from build123d import *

# Parameters (mm, degrees)
EXTRUDE_1_DEPTH     = 145
SKETCH_2_R          = 1.35
CUT_EXTRUDE_1_DEPTH = 3
CUT_EXTRUDE_2_DEPTH = 2.5
CUT_EXTRUDE_3_DEPTH = 70
FILLET_1_R          = 2.5
FILLET_2_R          = 1.5


with BuildPart() as part:
    # 草图1 → 凸台-拉伸1 (new body)
    with BuildSketch(Plane.XY):
        Polygon((-13, -35.966337082), (-13, -23.466337082), (40.5, -23.466337082), (40.5, -93.466337082), (-13, -93.466337082), (-13, -80.966337082), (-10, -80.966337082), (-10, -90.966337082), (38, -90.966337082), (38, -25.966337082), (-10, -25.966337082), (-10, -35.966337082), align=None)
    extrude(amount=-EXTRUDE_1_DEPTH)

    # 草图2 → 切除-拉伸1 (cut)
    with BuildSketch(Plane.ZY.offset(13)):
        with Locations((-112.5, -30.966337082)):
            Circle(SKETCH_2_R)
        with Locations((-72.5, -30.966337082)):
            Circle(SKETCH_2_R)
        with Locations((-32.5, -30.966337082)):
            Circle(SKETCH_2_R)
        with Locations((-32.5, -85.966337082)):
            Circle(SKETCH_2_R)
        with Locations((-72.5, -85.966337082)):
            Circle(SKETCH_2_R)
        with Locations((-112.5, -85.966337082)):
            Circle(SKETCH_2_R)
    extrude(amount=-CUT_EXTRUDE_1_DEPTH, mode=Mode.SUBTRACT)

    # 草图3 → 切除-拉伸2 (cut)
    with BuildSketch(Plane.ZY.offset(-38)):
        with BuildLine():
            Line((-128, -33.466337082), (-83, -33.466337082))
            ThreePointArc((-83, -33.466337082), (-78, -38.466337082), (-83, -43.466337082))
            Line((-83, -43.466337082), (-128, -43.466337082))
            ThreePointArc((-128, -43.466337082), (-133, -38.466337082), (-128, -33.466337082))
        make_face()
        with BuildLine():
            Line((-128, -53.466337082), (-83, -53.466337082))
            ThreePointArc((-83, -53.466337082), (-78, -58.466337082), (-83, -63.466337082))
            Line((-83, -63.466337082), (-128, -63.466337082))
            ThreePointArc((-128, -63.466337082), (-133, -58.466337082), (-128, -53.466337082))
        make_face()
        with BuildLine():
            Line((-128, -73.466337082), (-83, -73.466337082))
            ThreePointArc((-83, -73.466337082), (-78, -78.466337082), (-83, -83.466337082))
            Line((-83, -83.466337082), (-128, -83.466337082))
            ThreePointArc((-128, -83.466337082), (-133, -78.466337082), (-128, -73.466337082))
        make_face()
        with BuildLine():
            Line((-60, -33.466337082), (-15, -33.466337082))
            ThreePointArc((-15, -33.466337082), (-10, -38.466337082), (-15, -43.466337082))
            Line((-15, -43.466337082), (-60, -43.466337082))
            ThreePointArc((-60, -43.466337082), (-65, -38.466337082), (-60, -33.466337082))
        make_face()
        with BuildLine():
            Line((-60, -53.466337082), (-15, -53.466337082))
            ThreePointArc((-15, -53.466337082), (-10, -58.466337082), (-15, -63.466337082))
            Line((-15, -63.466337082), (-60, -63.466337082))
            ThreePointArc((-60, -63.466337082), (-65, -58.466337082), (-60, -53.466337082))
        make_face()
        with BuildLine():
            Line((-60, -73.466337082), (-15, -73.466337082))
            ThreePointArc((-15, -73.466337082), (-10, -78.466337082), (-15, -83.466337082))
            Line((-15, -83.466337082), (-60, -83.466337082))
            ThreePointArc((-60, -83.466337082), (-65, -78.466337082), (-60, -73.466337082))
        make_face()
    extrude(amount=-CUT_EXTRUDE_2_DEPTH, mode=Mode.SUBTRACT)

    # 草图4 → 切除-拉伸3 (cut)
    with BuildSketch(Plane(origin=(0, -23.466337082, 0), x_dir=(1, 0, 0), z_dir=(0, 1, 0))):
        Polygon((28.75, 85.438393953), (-1.25, 72.5), (28.75, 59.561606047), align=None)
        Polygon((-1.25, 127.5), (28.75, 114.561606047), (28.75, 127.5), align=None)
        Polygon((-1.25, 112.938393953), (28.75, 100), (-1.25, 87.061606047), align=None)
        Polygon((-1.25, 57.938393953), (28.75, 45), (-1.25, 32.061606047), align=None)
        Polygon((-1.25, 17.5), (28.75, 30.438393953), (28.75, 17.5), align=None)
    extrude(amount=-CUT_EXTRUDE_3_DEPTH, mode=Mode.SUBTRACT)

    # 圆角1
    fillet_1_edges = [part.edges().sort_by_distance(p)[0] for p in [
        (-1.25, -92.216337082, -127.5),
        (28.75, -92.216337082, -127.5),
        (28.75, -92.216337082, -114.561606047),
        (-1.25, -24.716337082, -127.5),
        (28.75, -24.716337082, -127.5),
        (28.75, -24.716337082, -114.561606047),
        (-1.25, -92.216337082, -32.061606047),
        (-1.25, -92.216337082, -57.938393953),
        (28.75, -92.216337082, -45),
        (-1.25, -24.716337082, -32.061606047),
        (-1.25, -24.716337082, -57.938393953),
        (28.75, -24.716337082, -45),
        (-1.25, -92.216337082, -87.061606047),
        (-1.25, -92.216337082, -112.938393953),
        (28.75, -92.216337082, -100),
        (-1.25, -24.716337082, -87.061606047),
        (-1.25, -24.716337082, -112.938393953),
        (28.75, -24.716337082, -100),
        (28.75, -92.216337082, -85.438393953),
        (28.75, -92.216337082, -59.561606047),
        (-1.25, -92.216337082, -72.5),
        (28.75, -24.716337082, -85.438393953),
        (28.75, -24.716337082, -59.561606047),
        (-1.25, -24.716337082, -72.5),
        (28.75, -92.216337082, -17.5),
        (-1.25, -92.216337082, -17.5),
        (28.75, -92.216337082, -30.438393953),
        (28.75, -24.716337082, -17.5),
        (-1.25, -24.716337082, -17.5),
        (28.75, -24.716337082, -30.438393953),
    ]]
    fillet(fillet_1_edges, radius=FILLET_1_R)

    # 圆角2
    fillet_2_edges = [part.edges().sort_by_distance(p)[0] for p in [
        (-13, -23.466337082, -72.5),
        (40.5, -23.466337082, -72.5),
        (40.5, -93.466337082, -72.5),
        (-13, -93.466337082, -72.5),
        (-10, -90.966337082, -72.5),
        (38, -90.966337082, -72.5),
        (38, -25.966337082, -72.5),
        (-10, -25.966337082, -72.5),
    ]]
    fillet(fillet_2_edges, radius=FILLET_2_R)


solid = part.part
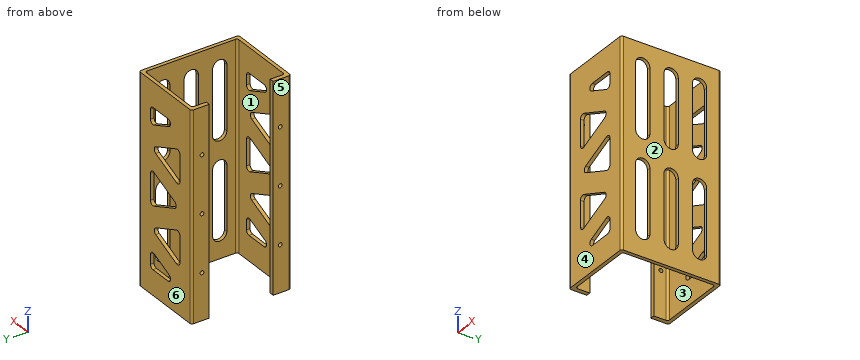
CAD build for the part. Positions are in the model's coordinates, mm. Face numbers are marked on the shaded views. A direction names the side the tool comes from. Give positions to 0.01 mm unless a question says otherwise; leave off trailing zeros. Order: outer loops, then holes, each group sorted by start corner. A loop starts at its lowest first (then second) coordinate and runs counter-clockwise, first axis right, second up. Notation, with made-up numbers: (45, -17) -> (85, -17) arc R17 cw to (85, -8) -> close; hole circle Ø6 at (55, 59.25). An arc over 180 degrees is marked (long way). Return JSON: item names as keys, results as strings.
Q1. Drill centre lines: line 1 (Y direction, x = -11, z = -72.5); line 2 (Y direction, x = -3.5, z = -46); line 3 (Y direction, x = -12, z = -72.5). Where is each one in solid material? Low to high.
Working result:
{"line 1": "-93.47 to -87.32, -84.62 to -80.97, -35.97 to -32.32, -29.62 to -23.47", "line 2": "-93.47 to -90.97, -25.97 to -23.47", "line 3": "-93.38 to -87.32, -84.62 to -80.97, -35.97 to -32.32, -29.62 to -23.55"}
Q2. Saw through at C-C (z = -135). Write the cut outline in (x, y), then the cut area to 3 significant figures.
Working result:
{"outline": "(-13, -91.97) arc R1.5 ccw to (-11.5, -93.47) -> (39, -93.47) arc R1.5 ccw to (40.5, -91.97) -> (40.5, -24.97) arc R1.5 ccw to (39, -23.47) -> (-11.5, -23.47) arc R1.5 ccw to (-13, -24.97) -> (-13, -35.97) -> (-10, -35.97) -> (-10, -27.47) arc R1.5 cw to (-8.5, -25.97) -> (36.5, -25.97) arc R1.5 cw to (38, -27.47) -> (38, -89.47) arc R1.5 cw to (36.5, -90.97) -> (-8.5, -90.97) arc R1.5 cw to (-10, -89.47) -> (-10, -80.97) -> (-13, -80.97) -> close", "area": "490 mm²"}
Q3. Saw through at A-A (x = -4). Write the cut outline in (y, z).
Working result:
{"outline": "(-93.47, -145) -> (-90.97, -145) -> (-90.97, 0) -> (-93.47, 0) -> close; (-25.97, -145) -> (-23.47, -145) -> (-23.47, 0) -> (-25.97, 0) -> close"}
Q4. Flat gauge pin, fed straight in: pin 1 (10 mm diameter, centred on y = -63.5, z = -72, fed in from -X). Where does the tip first touch, or does it go through?
Working result:
{"pin 1": "x = 38"}
Q5. Saw through at D-D (z = -104). Count the separate pieces of the cut face and the enclosed holes in it, then the cut area to 3 significant figures.
Working result:
{"separate pieces": "6", "enclosed holes": "0", "area": "311 mm²"}
Q6. Mould opens along Y. For the marked faces 3, 4, 5 and 6 say: pulls with the +Y half, pulls with the -Y half, needs draft (parallel to the pull), parting line crosses it, or undercut.
Working result:
{"face 3": "undercut", "face 4": "pulls with the -Y half", "face 5": "needs draft", "face 6": "pulls with the +Y half"}
Q7. Saw through at B-B (y = -78). Write the cut outline in (x, z), then the cut area to 3 significant figures.
Working result:
{"outline": "(38, -145) -> (40.5, -145) -> (40.5, -132.98) -> (38, -132.98) -> close; (38, -78.02) -> (40.5, -78.02) -> (40.5, -64.98) -> (38, -64.98) -> close; (38, -10.02) -> (40.5, -10.02) -> (40.5, 0) -> (38, 0) -> close", "area": "87.7 mm²"}
Q8. Which spindle directions (+Z, -Z, +X, -X, +Y, -Y) get a long thin tool onto all of the face, cutting with end or side? Do the marked faces 1 and 2. Say none if no direction does.
Working result:
{"face 1": "+Z, -Z", "face 2": "+Z, -Z, +X, +Y, -Y"}
